from build123d import *

# Parameters (mm, degrees)
F0_W     = 584.2
F0_H     = 219.71
F1_DEPTH = 5.334
F2_W     = 571.5
F2_H     = 213.36
F2_W_2   = 546.1
F2_H_2   = 187.96
F3_DEPTH = 12.7
F4_R     = 25.4
F6_DEPTH = 12.7
F8_DEPTH = 5.334


# Not quite as in the source:
# - a feature names something its author has since deleted; it is built from what else it names


with BuildPart() as f1:
    # F0 (on Front) → F1 (new body)
    with BuildSketch(Plane.XZ):
        with Locations((-292.1, 109.855)):
            Rectangle(F0_W, F0_H)
    extrude(amount=F1_DEPTH)

    # F2 (on face) → F3 (join)
    with BuildSketch(Plane.XZ.offset(5.334)):
        with Locations((-292.1, 113.03)):
            Rectangle(F2_W, F2_H)
        with Locations((-292.1, 113.03)):
            Rectangle(F2_W_2, F2_H_2, mode=Mode.SUBTRACT)
    extrude(amount=F3_DEPTH)

    # F4
    f4_edges = [f1.edges().sort_by_distance(p)[0] for p in [
        (-565.15, -11.684, 207.01),
        (-19.05, -11.684, 207.01),
        (-19.05, -11.684, 19.05),
        (-565.15, -11.684, 19.05),
    ]]
    fillet(f4_edges, radius=F4_R)

    # F5 (on face) → F6 (cut)
    with BuildSketch(Plane.XZ.offset(18.034)):
        Polygon((-118.11, 219.71), (-125.73, 207.01), (-118.11, 207.01), (-113.5820166854, 214.5566388576), (-110.49, 219.71), align=None)
        Polygon((-56.5979833146, 214.5566388576), (-52.07, 207.01), (-44.45, 207.01), (-52.07, 219.71), (-59.69, 219.71), align=None)
        Polygon((-59.69, 219.71), (-110.49, 219.71), (-113.5820166854, 214.5566388576), (-56.5979833146, 214.5566388576), align=None)
    extrude(amount=-F6_DEPTH, mode=Mode.SUBTRACT)

    # F7 (on face) → F8 (join)
    with BuildSketch(Plane(origin=(0, 0, 0), x_dir=(-1, 0, 0), z_dir=(0, 1, 0))):
        Polygon((-5.08, 0), (0, 0), (0, 219.71), align=None)
        Polygon((584.2, 219.71), (584.2, 0), (589.28, 0), align=None)
        with BuildLine():
            Line((-5.08, 229.87), (0, 219.71))
            Line((0, 219.71), (148.0852009026, 219.71))
            add(Edge.make_bspline(
                [(148.0852009026, 219.71), (115.3779899576, 221.1840971885), (80.5489949788, 225.5270485943), (45.72, 229.87)],
                knots=[0.812101374, 0.812101374, 0.812101374, 0.812101374, 1, 1, 1, 1], degree=3))
            Line((45.72, 229.87), (-5.08, 229.87))
        make_face()
        with BuildLine():
            Line((436.1147990974, 219.71), (584.2, 219.71))
            Line((584.2, 219.71), (589.28, 229.87))
            Line((589.28, 229.87), (538.48, 229.87))
            add(Edge.make_bspline(
                [(538.48, 229.87), (503.6510050212, 225.5270485943), (468.8220100424, 221.1840971885), (436.1147990974, 219.71)],
                knots=[0, 0, 0, 0, 0.187898626, 0.187898626, 0.187898626, 0.187898626], degree=3))
        make_face()
        with BuildLine():
            add(Edge.make_bspline(
                [(292.1, 229.87), (259.7414000619, 229.87), (227.3828001238, 221.731425099), (190.5, 219.71)],
                knots=[0.5, 0.5, 0.5, 0.5, 0.7280781407, 0.7280781407, 0.7280781407, 0.7280781407], degree=3))
            Line((190.5, 219.71), (393.7, 219.71))
            add(Edge.make_bspline(
                [(393.7, 219.71), (356.8171998762, 221.731425099), (324.4585999381, 229.87), (292.1, 229.87)],
                knots=[0.2719218593, 0.2719218593, 0.2719218593, 0.2719218593, 0.5, 0.5, 0.5, 0.5], degree=3))
        make_face()
    extrude(amount=-F8_DEPTH)


solid = f1.part
Model file for the job. Use its own axes, mm. A direction names the side the tool comes from. Give positions to 0.01 mm unless a question says otherwise; leave off trailing zeros. Loops run counter-clockwise (first coordinate to the right, second up) from the corner with the lowest first, then second, coordinate; pieces in that order, holes last.
1) Tool access for faces 1 (the flat face through (-577.85, -12, 112)), 2 (the flat face through (-86, -12, 207.01)), 3 (the flat face through (-30, -12, 219.71)), 4 (the flat face through (-296, -12, 6.35)): list every direction of +Z, -Z, +X, -X, +Y, -Y with a clear straight run to the whole face (end or side of a thin tool).
2) Wall check: line 1 (X direction, y = -9, z = 152); line 2 (Z direction, x = -196, y = -8.75); line 3 (Z direction, x = -79, y = -6.5). Give the ranges that are in metal, low to high.
3) Saw through at B-B (x = -177). Write the cut outline in (y, z), plus the area to 3 significant figures.
4) Flat gauge pins, fed straight in: pin 1 Ø8 at (y, z) = (-14.5, 171) entering from -X; pin 2 Ø4 at (x, y) = (-80.5, -12) entering from -Z; pin 3 Ø4 at (x, y) = (-35, -14.5) entering from +Z. Where does each tip first touch, or does it go through?
5) Pull direction X, two halves, no side cores. Call faces 5 (the flat face through (-6.35, -12, 112)), 6 (the flat face through (-85, -12, 214.557)), 7 (the flat face through (-48.207, -11.773, 213.271)), 8 (the flat face through (-288, 0, 121)): +X half, -X half, draft (parallel to the pull), parting line (faces both ways), or undercut.
6) Saw through at D-D (z = 200.5). Write the cut outline in (x, y), plus the area to 3 significant figures.
7) Saw through at A-A (y = -8.75). Write the cut outline in (x, z).
8) Saw through at C-C (z = 133.5). Write the cut outline in (x, y), plus the area to 3 significant figures.
Answer block:
1. face 1: +Z, -Z, -X, -Y
1. face 2: -Y
1. face 3: +Z, +X, -X, -Y
1. face 4: -Z, +X, -X, -Y
2. line 1: x = -577.85 to -565.15, -19.05 to -6.35
2. line 2: z = 6.35 to 19.05, 207.01 to 219.71
2. line 3: z = 6.35 to 19.05, 207.01 to 214.56
3. outline: (-18.03, 6.35) - (-5.33, 6.35) - (-5.33, 0) - (0, 0) - (0, 219.71) - (-18.03, 219.71) - (-18.03, 207.01) - (-5.33, 207.01) - (-5.33, 19.05) - (-18.03, 19.05) - close
3. area: 1,490 mm2
4. pin 1: stops at x = -577.85
4. pin 2: stops at z = 6.35
4. pin 3: stops at z = 219.71
5. face 5: +X half
5. face 6: undercut
5. face 7: undercut
5. face 8: draft
6. outline: (-584.64, -5.33) - (-577.85, -5.33) - (-577.85, -18.03) - (-556.73, -18.03) - (-556.73, -5.33) - (-27.47, -5.33) - (-27.47, -18.03) - (-6.35, -18.03) - (-6.35, -5.33) - (0.44, -5.33) - (0.44, 0) - (-584.64, 0) - close
6. area: 3,660 mm2
7. outline: (-577.85, 6.35) - (-6.35, 6.35) - (-6.35, 219.71) - (-52.07, 219.71) - (-44.45, 207.01) arc R25.4 cw to (-19.05, 181.61) - (-19.05, 44.45) arc R25.4 cw to (-44.45, 19.05) - (-539.75, 19.05) arc R25.4 cw to (-565.15, 44.45) - (-565.15, 181.61) arc R25.4 cw to (-539.75, 207.01) - (-125.73, 207.01) - (-118.11, 219.71) - (-577.85, 219.71) - close; (-118.11, 207.01) - (-52.07, 207.01) - (-56.6, 214.56) - (-113.58, 214.56) - close
8. outline: (-586.19, -5.33) - (-577.85, -5.33) - (-577.85, -18.03) - (-565.15, -18.03) - (-565.15, -5.33) - (-19.05, -5.33) - (-19.05, -18.03) - (-6.35, -18.03) - (-6.35, -5.33) - (1.99, -5.33) - (1.99, 0) - (-586.19, 0) - close
8. area: 3,460 mm2
